from build123d import *

# Parameters (mm, degrees)
F0_W     = 101.6
F0_H     = 76.2
F1_DEPTH = 152.4
F2_W     = 76.2
F2_H     = 25.4
F3_DEPTH = 65.786
F4_R     = 6.132102


with BuildPart() as f1:
    # F0 (on Top) → F1 (new body)
    with BuildSketch(Plane.XY):
        with Locations((-10.087167, 2.012966)):
            Rectangle(F0_W, F0_H)
    extrude(amount=F1_DEPTH)

    # F2 (on face) → F3 (cut)
    with BuildSketch(Plane.XZ.offset(36.087034)):
        with Locations((-10.087167, 129.54)):
            Rectangle(F2_W, F2_H)
        with Locations((-10.087167, 93.98)):
            Rectangle(F2_W, F2_H)
        with Locations((-10.087167, 58.42)):
            Rectangle(F2_W, F2_H)
        with Locations((-10.087167, 22.86)):
            Rectangle(F2_W, F2_H)
    extrude(amount=-F3_DEPTH, mode=Mode.SUBTRACT)

    # F4
    f4_edges = [f1.edges().sort_by_distance(p)[0] for p in [
        (-60.887167, 2.012966, 152.4),
        (-10.087167, -36.087034, 152.4),
        (40.712833, 2.012966, 152.4),
        (-10.087167, 40.112966, 152.4),
        (40.712833, -36.087034, 76.2),
        (40.712833, 40.112966, 76.2),
        (-60.887167, 40.112966, 76.2),
        (-60.887167, -36.087034, 76.2),
        (-10.087167, -36.087034, 0),
        (-10.087167, 40.112966, 0),
        (40.712833, 2.012966, 0),
        (-60.887167, 2.012966, 0),
    ]]
    fillet(f4_edges, radius=F4_R)


solid = f1.part
Check sheet for the modelled part. Datum: model origin and axes. Units: mm. A direction names the side the tool comes from. Round coordinates to 2 decimals unless told otherwise and drop trailing zeros. Loops run counter-clockwise (first coordinate to the right, second up) from the corner with the lowest first, then second, coordinate; pieces in that order, holes last. Notation, with made-up numbers: (-37, 76.5) - (19, 76.5) arc R21 cw to (19, 96.5) - close; hole circle Ø2 at (-5, 6.5). An arc over 180 degrees is marked (long way). Answer as CSV lines item,"result". Start each with the question number.
Item 1: Section check B-B (z = 87). Record the boundary of the cut face in (x, y), and give its area (3 significant figures).
Item 2: Section check A-A (y = -6.5). Record the boundary of the cut face in (x, z).
Item 3: Depth check by flat-ended pin: P1, Ø20.5, axis at x = -7, z = 59.5, coming from the -Y side. Enter the tip coordinate at first touch or a pass-through.
Item 4: Release check for a two-part mould opening along X. For faces 3 (the flat face through (-11, -4, 81.28)), 4 (the flat face through (-11, 2, 152.4)), 5 (the flat face through (-48.187, -4, 94)), 6 (the cylindrical face through (-59.14, -34.24, 77.18)) record: +X half, -X half, draft (parallel to the pull), parting line (faces both ways), or undercut.
Item 5: Scan lines: line 1 (Z direction, x = 19.5, y = -27); line 2 (X direction, y = -12.5, z = 100.5); line 3 (Y direction, x = 2, z = 22). Record each from-to range of solid material in increasing order. Write a range as [from, to].
Item 6: Section check C-C (x = 6). Record the boundary of the cut face in (y, z).
Item 7: Set-up check for faces 1 (the flat face through (-11, 40.113, 75)), 2 (the flat face through (-11, -4, 116.84)): record each of +Z, -Z, +X, -X, +Y, -Y from which the full face is reachable in a straight line by a thin tool's end or side.
Report:
1,outline,"(-60.89, -29.95) arc R6.13 ccw to (-54.76, -36.09) - (-48.19, -36.09) - (-48.19, 29.7) - (28.01, 29.7) - (28.01, -36.09) - (34.58, -36.09) arc R6.13 ccw to (40.71, -29.95) - (40.71, 33.98) arc R6.13 ccw to (34.58, 40.11) - (-54.76, 40.11) arc R6.13 ccw to (-60.89, 33.98) - close"
1,area,"2,700 mm2"
2,outline,"(-60.89, 6.13) arc R6.13 ccw to (-54.76, 0) - (34.58, 0) arc R6.13 ccw to (40.71, 6.13) - (40.71, 146.27) arc R6.13 ccw to (34.58, 152.4) - (-54.76, 152.4) arc R6.13 ccw to (-60.89, 146.27) - close; hole (-48.19, 10.16) - (28.01, 10.16) - (28.01, 35.56) - (-48.19, 35.56) - close; hole (-48.19, 45.72) - (28.01, 45.72) - (28.01, 71.12) - (-48.19, 71.12) - close; hole (-48.19, 81.28) - (28.01, 81.28) - (28.01, 106.68) - (-48.19, 106.68) - close; hole (-48.19, 116.84) - (28.01, 116.84) - (28.01, 142.24) - (-48.19, 142.24) - close"
3,P1,"stops at y = 29.7"
4,face 3,"undercut"
4,face 4,"draft"
4,face 5,"undercut"
4,face 6,"-X half"
5,line 1,"z = [0, 10.16], [35.56, 45.72], [71.12, 81.28], [106.68, 116.84], [142.24, 152.4]"
5,line 2,"x = [-60.89, -48.19], [28.01, 40.71]"
5,line 3,"y = [29.7, 40.11]"
6,outline,"(-36.09, 6.13) arc R6.13 ccw to (-29.95, 0) - (33.98, 0) arc R6.13 ccw to (40.11, 6.13) - (40.11, 146.27) arc R6.13 ccw to (33.98, 152.4) - (-29.95, 152.4) arc R6.13 ccw to (-36.09, 146.27) - (-36.09, 142.24) - (29.7, 142.24) - (29.7, 116.84) - (-36.09, 116.84) - (-36.09, 106.68) - (29.7, 106.68) - (29.7, 81.28) - (-36.09, 81.28) - (-36.09, 71.12) - (29.7, 71.12) - (29.7, 45.72) - (-36.09, 45.72) - (-36.09, 35.56) - (29.7, 35.56) - (29.7, 10.16) - (-36.09, 10.16) - close"
7,face 1,"+Z, -Z, +X, -X, +Y"
7,face 2,"-Y"
